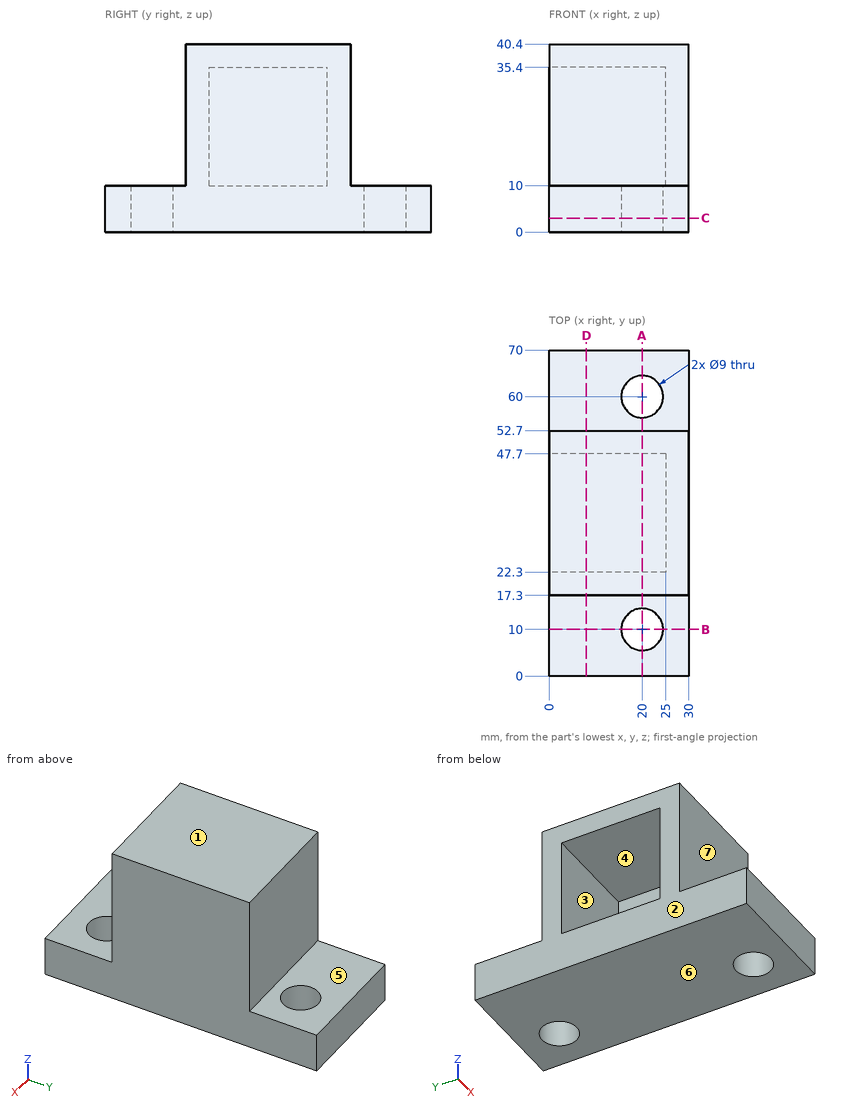
Verification items for this drawing (mm, ordinates from the low corner). A direction names the side the tool comes from. Round coordinates to 2 decimals unless told otherwise and drop trailing zeros. Write each loop counter-clockwise with the first axis right and the second up, starting at its lowest first coordinate (ties: lowest second). Pieces come first, ordered by that corner, then holes. Notation, with made-up numbers: (-4.75, -18.75) - (35.25, -18.75) arc R5 cw to (35.25, -9.75) - close; hole circle Ø10 at (-30.75, 1). An arc over 180 degrees is marked (long way). One line per item, written item: value.
1. Scan lines: L1, parallel to Y at x = 20, z = 7.75; L2, parallel to Y at x = 11, z = 28; L3, parallel to Z at x = 5.75, y = 33.5. Record each from-to range of solid material in increasing order.
The answers:
L1: y = 0 to 5.5, 14.5 to 55.5, 64.5 to 70
L2: y = 17.3 to 22.3, 47.7 to 52.7
L3: z = 0 to 10, 35.4 to 40.4
2. Cross-section at B-B on y = 10. Record the boundary of the cut face in (x, z).
The answers:
outline: (0, 0) - (15.5, 0) - (15.5, 10) - (0, 10) - close; (24.5, 0) - (30, 0) - (30, 10) - (24.5, 10) - close
3. Mould release check, pull along Z, two halves, no side actions. Record for the marked faces 1, 2, 3 and 4: released by +Z, released by -Z, zero draft, split by the parting line, or undercut.
The answers:
face 1: released by +Z
face 2: zero draft
face 3: undercut
face 4: undercut
4. Set-up check for the marked faces 5, 6 and 7: record each of +Z, -Z, +X, -X, +Y, -Y from which the full face is reachable in a straight line by a thin tool's end or side.
The answers:
face 5: +Z, +X, -X, +Y
face 6: -Z, +X, -X, +Y, -Y
face 7: +Z, +X, -X, -Y
5. Depth check by flat-ended pin: pin 1 Ø6 at (x, z) = (5, 13.5) entering from -Y; pin 2 Ø5 at (x, y) = (22.5, 11.5) entering from +Z; pin 3 Ø5 at (x, z) = (19, 30.5) entering from +Y; pin 4 Ø7 at (x, y) = (20, 10) entering from -Z. Enter the tip coordinate at first touch or a pass-through.
The answers:
pin 1: stops at y = 17.3
pin 2: stops at z = 10
pin 3: stops at y = 52.7
pin 4: passes through
6. Cross-section at A-A on x = 20. Record the boundary of the cut face in (y, z), and give its area (3 significant figures).
The answers:
outline: (0, 0) - (5.5, 0) - (5.5, 10) - (0, 10) - close; (14.5, 0) - (55.5, 0) - (55.5, 10) - (52.7, 10) - (52.7, 40.4) - (17.3, 40.4) - (17.3, 10) - (14.5, 10) - close; (64.5, 0) - (70, 0) - (70, 10) - (64.5, 10) - close; hole (22.3, 10) - (47.7, 10) - (47.7, 35.4) - (22.3, 35.4) - close
area: 951 mm^2
7. Cross-section at C-C on z = 3. Record the boundary of the cut face in (x, y), and give its area (3 significant figures).
The answers:
outline: (0, 0) - (30, 0) - (30, 70) - (0, 70) - close; hole circle Ø9 at (20, 10); hole circle Ø9 at (20, 60)
area: 1,970 mm^2
8. Cross-section at D-D on x = 8. Record the boundary of the cut face in (y, z).
The answers:
outline: (0, 0) - (70, 0) - (70, 10) - (52.7, 10) - (52.7, 40.4) - (17.3, 40.4) - (17.3, 10) - (0, 10) - close; hole (22.3, 10) - (47.7, 10) - (47.7, 35.4) - (22.3, 35.4) - close
